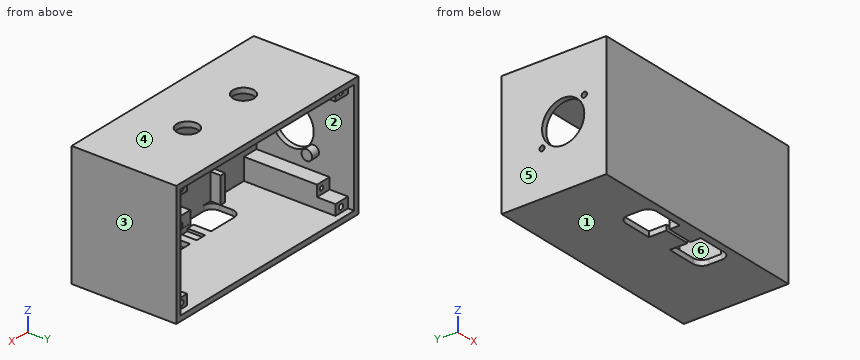
```python
from build123d import *

# Parameters (mm, degrees)
SKETCH1_W       = 130
SKETCH1_H       = 70
EXTRUDE1_DEPTH  = 4
SKETCH2_W       = 130
SKETCH2_H       = 70
SKETCH2_W_2     = 124
SKETCH2_H_2     = 64
EXTRUDE2_DEPTH  = 55.5
SKETCH3_W       = 15
SKETCH3_H       = 1.7
EXTRUDE3_DEPTH  = 4.8
SKETCH4_W       = 3
SKETCH4_H       = 15
EXTRUDE5_DEPTH  = 5.8
SKETCH5_W       = 6
SKETCH5_H       = 10.139345217
EXTRUDE6_DEPTH  = 1.5
SKETCH22_R      = 3
EXTRUDE26_DEPTH = 8
SKETCH10_R      = 12
SKETCH10_R_2    = 1.5
EXTRUDE11_DEPTH = 6
EXTRUDE13_START = -3.5
SKETCH12_W      = 9
SKETCH12_H      = 6
EXTRUDE13_DEPTH = 52
EXTRUDE14_START = -3.5
SKETCH13_W      = 9
SKETCH13_H      = 6
EXTRUDE14_DEPTH = 52
SKETCH14_R      = 1.55
EXTRUDE15_DEPTH = 8
SKETCH20_R      = 1.55
EXTRUDE22_DEPTH = 8
SKETCH23_W      = 9
SKETCH23_H      = 6.3
EXTRUDE27_DEPTH = 41.5
SKETCH24_R      = 6.1
EXTRUDE28_DEPTH = 5
SKETCH25_R      = 1.25
EXTRUDE29_DEPTH = 8


with BuildPart() as part:
    # Sketch1 → Extrude1 (new body)
    with BuildSketch(Plane(origin=(0, 0, 0), x_dir=(1, 0, 0), z_dir=(0, 1, 0))):
        Rectangle(SKETCH1_W, SKETCH1_H)
    extrude(amount=EXTRUDE1_DEPTH)

    # Sketch2 → Extrude2 (add)
    with BuildSketch(Plane(origin=(0, 4, 0), x_dir=(1, 0, 0), z_dir=(0, 1, 0))):
        Rectangle(SKETCH2_W, SKETCH2_H)
        Rectangle(SKETCH2_W_2, SKETCH2_H_2, mode=Mode.SUBTRACT)
    extrude(amount=EXTRUDE2_DEPTH)

    # Sketch3 → Extrude3 (cut)
    with BuildSketch(Plane(origin=(0, 0, -35), x_dir=(-1, 0, 0), z_dir=(0, 0, -1))):
        with BuildLine():
            Line((-24, 21.6), (-7.5, 21.6))
            Line((-7.5, 21.6), (-7.5, 4))
            Line((-7.5, 4), (-24, 4))
            ThreePointArc((-24, 4), (-27.535533906, 5.464466094), (-29, 9))
            Line((-29, 9), (-29, 16.6))
            ThreePointArc((-29, 16.6), (-27.535533906, 20.135533906), (-24, 21.6))
        make_face()
        with BuildLine():
            Line((7.5, 4), (24, 4))
            ThreePointArc((24, 4), (27.535533906, 5.464466094), (29, 9))
            Line((29, 9), (29, 16.6))
            ThreePointArc((29, 16.6), (27.535533906, 20.135533906), (24, 21.6))
            Line((24, 21.6), (7.5, 21.6))
            Line((7.5, 21.6), (7.5, 4))
        make_face()
        with Locations((0, 10.75)):
            Rectangle(SKETCH3_W, SKETCH3_H)
    extrude(amount=-EXTRUDE3_DEPTH, mode=Mode.SUBTRACT)

    # Sketch4 → Extrude5 (add)
    with BuildSketch(Plane(origin=(0, 4, 0), x_dir=(1, 0, 0), z_dir=(0, 1, 0))):
        with BuildLine():
            Line((-0.871779789, 32), (-7.4, 32))
            Line((-7.4, 32), (-7.4, 25.2))
            Line((-7.4, 25.2), (7.4, 25.2))
            Line((7.4, 25.2), (7.4, 32))
            Line((7.4, 32), (0.871779789, 32))
            ThreePointArc((0.871779789, 32), (1.694632641, 31.262177109), (2, 30.2))
            ThreePointArc((2, 30.2), (-1.062177109, 28.505367359), (-0.871779789, 32))
        make_face()
        with Locations((-30.65, 24.5)):
            Rectangle(SKETCH4_W, SKETCH4_H)
        with Locations((30.65, 24.5)):
            Rectangle(SKETCH4_W, SKETCH4_H)
    extrude(amount=EXTRUDE5_DEPTH)

    # Sketch5 → Extrude6 (cut)
    with BuildSketch(Plane.XY.offset(-32)):
        with Locations((0, 16.669672609)):
            Rectangle(SKETCH5_W, SKETCH5_H)
    extrude(amount=-EXTRUDE6_DEPTH, mode=Mode.SUBTRACT)

    # Sketch22 → Extrude26 (add)
    with BuildSketch(Plane.ZY.offset(65)):
        with Locations((-9.5, 36.5)):
            Circle(SKETCH22_R)
        with Locations((9.5, 12.5)):
            Circle(SKETCH22_R)
    extrude(amount=-EXTRUDE26_DEPTH)

    # Sketch10 → Extrude11 (cut)
    with BuildSketch(Plane.ZY.offset(65)):
        with Locations((0, 24.5)):
            Circle(SKETCH10_R)
        with Locations((-9.5, 36.5)):
            Circle(SKETCH10_R_2)
        with Locations((9.5, 12.5)):
            Circle(SKETCH10_R_2)
    extrude(amount=-EXTRUDE11_DEPTH, mode=Mode.SUBTRACT)

    # Sketch12 → Extrude13 (add)
    with BuildSketch(Plane(origin=(0, 59.5, 0), x_dir=(1, 0, 0), z_dir=(0, 1, 0)).offset(EXTRUDE13_START)):
        with Locations((-57.5, -29)):
            Rectangle(SKETCH12_W, SKETCH12_H)
        with Locations((57.5, -29)):
            Rectangle(SKETCH12_W, SKETCH12_H)
    extrude(amount=-EXTRUDE13_DEPTH)

    # Sketch13 → Extrude14 (add)
    with BuildSketch(Plane(origin=(0, 59.5, 0), x_dir=(1, 0, 0), z_dir=(0, 1, 0)).offset(EXTRUDE14_START)):
        with Locations((-57.5, 29)):
            Rectangle(SKETCH13_W, SKETCH13_H)
        with Locations((57.5, 29)):
            Rectangle(SKETCH13_W, SKETCH13_H)
    extrude(amount=-EXTRUDE14_DEPTH)

    # Sketch14 → Extrude15 (cut)
    with BuildSketch(Plane(origin=(0, 59.5, 0), x_dir=(1, 0, 0), z_dir=(0, 1, 0))):
        with Locations(Location((-57, 29, 0), (0, 0, 270))):
            Circle(SKETCH14_R)
        with Locations(Location((57, 29, 0), (0, 0, 270))):
            Circle(SKETCH14_R)
    extrude(amount=-EXTRUDE15_DEPTH, mode=Mode.SUBTRACT)

    # Sketch20 → Extrude22 (cut)
    with BuildSketch(Plane(origin=(0, 59.5, 0), x_dir=(1, 0, 0), z_dir=(0, 1, 0))):
        with Locations(Location((-57, -29, 0), (0, 0, 270))):
            Circle(SKETCH20_R)
        with Locations(Location((57, -29, 0), (0, 0, 270))):
            Circle(SKETCH20_R)
    extrude(amount=-EXTRUDE22_DEPTH, mode=Mode.SUBTRACT)

    # Sketch23 → Extrude27 (add)
    with BuildSketch(Plane(origin=(0, 4, 0), x_dir=(1, 0, 0), z_dir=(0, 1, 0))):
        with Locations((-57.5, 22.85)):
            Rectangle(SKETCH23_W, SKETCH23_H)
        with Locations((-57.5, -22.85)):
            Rectangle(SKETCH23_W, SKETCH23_H)
        with Locations((57.5, -22.85)):
            Rectangle(SKETCH23_W, SKETCH23_H)
        with Locations((57.5, 22.85)):
            Rectangle(SKETCH23_W, SKETCH23_H)
    extrude(amount=EXTRUDE27_DEPTH)

    # Sketch24 → Extrude28 (cut)
    with BuildSketch(Plane.XY.offset(35)):
        with Locations((-20, 30)):
            Circle(SKETCH24_R)
        with Locations((20, 30)):
            Circle(SKETCH24_R)
    extrude(amount=-EXTRUDE28_DEPTH, mode=Mode.SUBTRACT)

    # Sketch25 → Extrude29 (cut)
    with BuildSketch(Plane(origin=(0, 45.5, 0), x_dir=(1, 0, 0), z_dir=(0, 1, 0))):
        with Locations(Location((-56.25, 22.86, 0), (0, 0, 270))):
            Circle(SKETCH25_R)
        with Locations(Location((56.25, 22.86, 0), (0, 0, 270))):
            Circle(SKETCH25_R)
        with Locations(Location((-56.25, -22.86, 0), (0, 0, 270))):
            Circle(SKETCH25_R)
        with Locations(Location((56.25, -22.86, 0), (0, 0, 270))):
            Circle(SKETCH25_R)
    extrude(amount=-EXTRUDE29_DEPTH, mode=Mode.SUBTRACT)


solid = part.part
```
Geometry check sheet. Reference: the model listing, model coordinates, mm. Face numbers are marked on the shaded views. A direction names the side the tool comes from. Give positions to 0.01 mm unless a question says otherwise; leave off trailing zeros. Order: outer loops, then holes, each group sorted by start corner. A loop starts at its lowest first (then second) coordinate and runs counter-clockwise, first axis right, second up.
1. Thickness scan on L1, parallel to X at y = 54.45, z = -29; L2, parallel to Y at x = -61.5, z = -9.5; L3, parallel to Z at x = -29, y = 22.5. Record the ranges inside material, lowest first.
2. Section check B-B, the plane y = 44. Enter the section's corners in (x, z).
3. Section check A-A, the plane x = -12.5. Enter the section's corners in (y, z), and give its area (3 significant figures).
4. Section check D-D, the plane z = -9.5. Enter the section's corners in (x, y).
5. Access from +Z, -Z, +X, -X, +Y, -Y to the whole of each face (thin tool, end or side, straight path). Record for the marked faces 5 and 6.
6. Section check C-C, the plane x = 48. Enter the section's corners in (y, z).
7. Release check for a two-part mould opening along Z. For the marked faces 1, 2, 3 and 4 record: pulls with the +Z half, pulls with the -Z half, needs draft (parallel to the pull), parting line crosses it, or undercut.
8. Gauge pin test, flat ends, axial feed: pin 1 Ø4 at (x, z) = (1, -29) entering from +Y; pin 2 Ø3 at (x, z) = (-59.5, -22) entering from +Y; pin 3 Ø2 at (x, z) = (56.25, -22.86) entering from +Y. Record the tip position at first contact, or that the pin passes through.
Values follow:
1. L1: x = -65 to -58.55, -55.45 to -53, 53 to 55.45, 58.55 to 65
1. L2: y = 0 to 4, 33.5 to 35, 38 to 39.5
1. L3: z = -35 to -32, 32 to 35
2. outline: (-65, -35) - (65, -35) - (65, 35) - (-65, 35) - close; hole (-62, -19.7) - (-53, -19.7) - (-53, -32) - (53, -32) - (53, -19.7) - (62, -19.7) - (62, 19.7) - (53, 19.7) - (53, 32) - (-53, 32) - (-53, 19.7) - (-62, 19.7) - close; hole circle Ø2.5 at (-56.25, -22.86); hole circle Ø2.5 at (-56.25, 22.86); hole circle Ø2.5 at (56.25, -22.86); hole circle Ø2.5 at (56.25, 22.86)
3. outline: (0, -35) - (4, -35) - (4, 32) - (59.5, 32) - (59.5, 35) - (0, 35) - close; (21.6, -35) - (59.5, -35) - (59.5, -32) - (21.6, -32) - close
3. area: 560 mm2
4. outline: (-65, 0) - (65, 0) - (65, 59.5) - (62, 59.5) - (62, 4) - (-62, 4) - (-62, 17.17) - (-65, 17.17) - close; (-65, 31.83) - (-62, 31.83) - (-62, 33.5) - (-57, 33.5) - (-57, 39.5) - (-62, 39.5) - (-62, 59.5) - (-65, 59.5) - (-65, 38) - (-59, 38) - (-59, 35) - (-65, 35) - close
5. face 5: +Z, -Z, -X, +Y, -Y
5. face 6: +Y
6. outline: (0, -35) - (59.5, -35) - (59.5, -32) - (4, -32) - (4, 32) - (59.5, 32) - (59.5, 35) - (0, 35) - close
7. face 1: pulls with the -Z half
7. face 2: undercut
7. face 3: needs draft
7. face 4: pulls with the +Z half
8. pin 1: stops at y = 9.8
8. pin 2: stops at y = 45.5
8. pin 3: stops at y = 37.5
